```python
from build123d import *

# Parameters (mm, degrees)
SKETCH1_W               = 106.68
SKETCH1_H               = 59.69
SKETCH1_W_2             = 101.6
SKETCH1_H_2             = 54.61
BOSS_EXTRUDE1_DEPTH     = 50.8
SKETCH2_W               = 106.68
SKETCH2_H               = 59.69
BOSS_EXTRUDE2_DEPTH     = 2.54
SKETCH3_R               = 2.032
CUT_EXTRUDE1_DEPTH      = 2.54
BOSS_EXTRUDE3_START     = -31.75
SKETCH5_W               = 15.24
SKETCH5_H               = 25.4
BOSS_EXTRUDE3_DEPTH     = 17.526
SKETCH6_W               = 13.97
SKETCH6_H               = 22.86
CUT_EXTRUDE2_DEPTH      = 23.114
SKETCH8_R               = 1.27
CUT_EXTRUDE3_DEPTH      = 122.833947508
FILLET3_R               = 2.54
SKETCH9_R               = 4.7625
BOSS_EXTRUDE4_DEPTH     = 3.175
SKETCH11_R              = 2.38125
CUT_EXTRUDE4_DEPTH      = 88.330393621
BOSS_EXTRUDE5_DEPTH     = 6.35
FILLET4_R               = 1.27
FILLET4_OF_MIRROR2_R    = 1.27
FILLET6_R               = 1.27
SKETCH14_W              = 13.97
SKETCH14_H              = 5.08
BOSS_EXTRUDE6_DEPTH     = 6.35
MIRROR6_COPY_1_SKETCH_W = 13.97
MIRROR6_COPY_1_SKETCH_H = 5.08
MIRROR6_COPY_1_DEPTH    = 6.35
CUT_EXTRUDE5_DEPTH      = 127
SKETCH15_R              = 4.826
BOSS_EXTRUDE7_DEPTH     = 3.175


with BuildPart() as part:
    # Sketch1 → Boss-Extrude1 (new body)
    with BuildSketch(Plane(origin=(0, 0, 0), x_dir=(1, 0, 0), z_dir=(0, 1, 0))):
        Rectangle(SKETCH1_W, SKETCH1_H)
        Rectangle(SKETCH1_W_2, SKETCH1_H_2, mode=Mode.SUBTRACT)
    extrude(amount=BOSS_EXTRUDE1_DEPTH)

    # Sketch2 → Boss-Extrude2 (add)
    with BuildSketch(Plane(origin=(0, 0, 0), x_dir=(-1, 0, 0), z_dir=(0, -1, 0))):
        Rectangle(SKETCH2_W, SKETCH2_H)
    extrude(amount=-BOSS_EXTRUDE2_DEPTH)

    # Sketch3 → Cut-Extrude1 (cut)
    with BuildSketch(Plane.XZ):
        with Locations(Location((-19.05, 19.05, 0), (0, 0, 270))):
            Circle(SKETCH3_R)
        with Locations(Location((19.05, 19.05, 0), (0, 0, 270))):
            Circle(SKETCH3_R)
        with Locations(Location((19.05, -19.05, 0), (0, 0, 270))):
            Circle(SKETCH3_R)
        with Locations(Location((-19.05, -19.05, 0), (0, 0, 270))):
            Circle(SKETCH3_R)
    extrude(amount=-CUT_EXTRUDE1_DEPTH, mode=Mode.SUBTRACT)

    # Sketch5 → Boss-Extrude3 (add)
    with BuildSketch(Plane.XZ.offset(BOSS_EXTRUDE3_START)):
        with Locations((-60.96, 0)):
            Rectangle(SKETCH5_W, SKETCH5_H)
    boss_extrude3 = extrude(amount=-BOSS_EXTRUDE3_DEPTH)

    # Sketch6 → Cut-Extrude2 (cut)
    with BuildSketch(Plane(origin=(0, 49.276, 0), x_dir=(1, 0, 0), z_dir=(0, 1, 0))):
        with Locations((-60.325, 0)):
            Rectangle(SKETCH6_W, SKETCH6_H)
    cut_extrude2 = extrude(amount=-CUT_EXTRUDE2_DEPTH, mode=Mode.SUBTRACT)

    # Sketch8 → Cut-Extrude3 (cut)
    with BuildSketch(Plane(origin=(-53.34, -47.057304482, -0.79669661), x_dir=(0, 0, 1), z_dir=(-1, 0, 0))):
        with Locations((-11.43, 59.69)):
            Circle(SKETCH8_R)
    extrude(amount=-CUT_EXTRUDE3_DEPTH, mode=Mode.SUBTRACT)

    # Fillet3
    fillet3_edges = [part.edges().sort_by_distance(p)[0] for p in [
        (-68.58, 40.513, -12.7),
        (-68.58, 40.513, 12.7),
    ]]
    fillet(fillet3_edges, radius=FILLET3_R)

    # Sketch9 → Boss-Extrude4 (add)
    with BuildSketch(Plane(origin=(0, 2.54, 0), x_dir=(1, 0, 0), z_dir=(0, 1, 0))):
        with Locations(Location((0, 0, 0), (0, 0, 270))):
            Circle(SKETCH9_R)
    extrude(amount=BOSS_EXTRUDE4_DEPTH)

    # Sketch11 → Cut-Extrude4 (cut, through all)
    with BuildSketch(Plane(origin=(0, 5.715, 0), x_dir=(1, 0, 0), z_dir=(0, 1, 0))):
        with Locations(Location((0, 0, 0), (0, 0, 270))):
            Circle(SKETCH11_R)
    extrude(amount=-CUT_EXTRUDE4_DEPTH, mode=Mode.SUBTRACT)

    # Sketch13 → Boss-Extrude5 (add, symmetric)
    with BuildSketch(Plane.XY):
        Polygon((-50.8, 46.99), (-48.26, 43.18), (-50.8, 43.18), align=None)
    boss_extrude5 = extrude(amount=BOSS_EXTRUDE5_DEPTH, both=True)

    # Fillet4
    fillet4_edges = [part.edges().sort_by_distance(p)[0] for p in [
        (-48.26, 43.18, 0),
    ]]
    fillet(fillet4_edges, radius=FILLET4_R)

    # Mirror2: Boss-Extrude5 across plane
    add(boss_extrude5.mirror(Plane(origin=(0, 0, 0), x_dir=(0, 0, 1), z_dir=(1, 0, 0))))

    # Fillet4 of Mirror2
    fillet4_of_mirror2_edges = [part.edges().sort_by_distance(p)[0] for p in [
        (48.26, 43.18, 0),
    ]]
    fillet(fillet4_of_mirror2_edges, radius=FILLET4_OF_MIRROR2_R)

    # Mirror4: Boss-Extrude3, Cut-Extrude2 across plane
    add(boss_extrude3.mirror(Plane(origin=(0, 0, 0), x_dir=(0, 0, 1), z_dir=(1, 0, 0))))
    add(cut_extrude2.mirror(Plane(origin=(0, 0, 0), x_dir=(0, 0, 1), z_dir=(1, 0, 0))), mode=Mode.SUBTRACT)

    # Fillet6
    fillet6_edges = [part.edges().sort_by_distance(p)[0] for p in [
        (68.58, 40.513, 12.7),
        (68.58, 40.513, -12.7),
    ]]
    fillet(fillet6_edges, radius=FILLET6_R)

    # Sketch14 → Boss-Extrude6 (add)
    with BuildSketch(Plane.XZ.offset(-31.75)):
        with Locations((-60.325, 15.24)):
            Rectangle(SKETCH14_W, SKETCH14_H)
    boss_extrude6 = extrude(amount=-BOSS_EXTRUDE6_DEPTH)

    # Mirror5: Boss-Extrude6 across plane
    add(boss_extrude6.mirror(Plane.XY))

    # Mirror6: Boss-Extrude6 across plane
    add(boss_extrude6.mirror(Plane(origin=(0, 0, 0), x_dir=(0, 0, 1), z_dir=(1, 0, 0))))

    # Mirror6 copy 1 sketch → Mirror6 copy 1 (add)
    with BuildSketch(Plane(origin=(0, 31.75, 0), x_dir=(-1, 0, 0), z_dir=(0, -1, 0))):
        with Locations((-60.325, 15.24)):
            Rectangle(MIRROR6_COPY_1_SKETCH_W, MIRROR6_COPY_1_SKETCH_H)
    extrude(amount=-MIRROR6_COPY_1_DEPTH)

    # Sketch12 → Cut-Extrude5 (cut, symmetric)
    with BuildSketch(Plane(origin=(0, 0, 0), x_dir=(0, 0, -1), z_dir=(1, 0, 0))):
        with BuildLine():
            Line((-29.845, 50.8), (-29.845, 44.694509634))
            ThreePointArc((-29.845, 44.694509634), (-25.725135532, 48.003392702), (-21.241724106, 50.8))
            Line((-21.241724106, 50.8), (-29.845, 50.8))
        make_face()
        with BuildLine():
            Line((29.845, 50.8), (21.241724106, 50.8))
            ThreePointArc((21.241724106, 50.8), (25.725135532, 48.003392702), (29.845, 44.694509634))
            Line((29.845, 44.694509634), (29.845, 50.8))
        make_face()
    extrude(amount=CUT_EXTRUDE5_DEPTH, both=True, mode=Mode.SUBTRACT)

    # Sketch15 → Boss-Extrude7 (add)
    with BuildSketch(Plane(origin=(0, 2.54, 0), x_dir=(1, 0, 0), z_dir=(0, 1, 0))):
        with Locations(Location((-29.21, 0, 0), (0, 0, 270))):
            Circle(SKETCH15_R)
        with Locations(Location((29.21, 0, 0), (0, 0, 270))):
            Circle(SKETCH15_R)
    extrude(amount=BOSS_EXTRUDE7_DEPTH)


solid = part.part
```
Geometry: final body of the model. Coordinates: model frame, mm. A direction names the side the tool comes from. Round coordinates to 2 decimals unless told otherwise and drop trailing zeros. Order: outer loops, then holes, each group sorted by start corner. A loop starts at its lowest first (then second) coordinate and runs counter-clockwise, first axis right, second up. Notation, with made-up numbers: (67, 41) - (100, 41) arc R19 cw to (100, 58) - close; hole circle Ø10 at (43.5, 71.25). An arc over 180 degrees is marked (long way). Write item = value, one per line. Start each with the question number.
Q1. Access query for faces 1 (the flat face through (60, 41, -11.43)), 2 (the flat face through (-29, 5.715, 0)), 3 (the flat face through (68, 31.75, 0)). Directions: +Z, -Z, +X, -X, +Y, -Y. A direction counts if a zero-diameter tool reaches every point of the face in a straight line with its end or side. Return the directions, or none.
Q2. Pin query (flat end, axial travel): pin 1 (6 mm diameter, centred on y = 33, z = 11, fed in from -X); pin 2 (4 mm diameter, centred on x = 63, y = 43.5, fed in from +Z); pin 3 (2.5 mm diameter, centred on y = 34, z = 14.5, fed in from +X); pin 4 (1.5 mm diameter, centred on y = 7.5, z = 6, fed in from +X). Return the tip coordinate at first contact, or that it passes through.
Q3. Cut plane A-A on z = -19.05. Return the cut outline in (x, y), and give its area (3 significant figures).
Q4. Pull-direction query (X, two-part tool) for faces 4 (the flat face through (60, 41, 11.43)), 5 (the flat face through (-68.58, 40, 0)), 6 (the flat face through (52, 50.8, 0)); classes: +X half, -X half, draft (parallel to the pull), parting line (faces both ways), or undercut.
Q5. Ray query, line 1 (X direction, y = 1.4, z = -19.05); line 2 (X direction, y = 20, z = 11); line 3 (Z direction, x = 9, y = 39) (3 decimals). Return the intervals inside material, ascending. Write a range as from..to.
Q6. Cut plane C-C on x = 19.05. Give the number of separate pieces and of enclosed holes in the cut face, and give its area (3 significant figures).
Outcome:
q1.face_1 = +Y, -Y
q1.face_2 = +Y
q1.face_3 = +Z, -Z, +X, -Y
q2.pin_1 = -68.58
q2.pin_2 = 12.7
q2.pin_3 = 67.31
q2.pin_4 = 53.34
q3.outline = (-53.34, 0) - (-21.08, 0) - (-21.08, 2.54) - (-50.8, 2.54) - (-50.8, 50.8) - (-53.34, 50.8) - close; (-17.02, 0) - (17.02, 0) - (17.02, 2.54) - (-17.02, 2.54) - close; (21.08, 0) - (53.34, 0) - (53.34, 50.8) - (50.8, 50.8) - (50.8, 2.54) - (21.08, 2.54) - close
q3.area = 495 mm^2
q4.face_4 = undercut
q4.face_5 = -X half
q4.face_6 = draft
q5.line_1 = -53.34..-21.08, -17.02..17.02, 21.08..53.34
q5.line_2 = -53.34..-50.8, 50.8..53.34
q5.line_3 = -29.845..-27.305, 27.305..29.845
q6.separate_pieces = 3
q6.enclosed_holes = 0
q6.area = 351 mm^2
